from build123d import *

# Parameters (mm, degrees)
F1_DEPTH = 25.4
F3_DEPTH = 12.7
F4_W     = 5.8812871575
F4_H     = 48.275558278
F4_W_2   = 5.8812852949
F5_DEPTH = 1.27
F7_DEPTH = 1.27


with BuildPart() as f1:
    # F0 (on Front) → F1 (new body)
    with BuildSketch(Plane.XZ):
        with BuildLine():
            Line((-42.643032968, 37.9803813994), (-42.643032968, 0))
            Line((-42.643032968, 0), (0, 0))
            Line((0, 0), (42.642146349, 0))
            Line((42.642146349, 0), (42.642146349, 37.9803813994))
            ThreePointArc((42.642146349, 37.9803813994), (-0.0004433095, 75.7243208105), (-42.643032968, 37.9803813994))
        make_face()
        Polygon((0, 0), (-42.643032968, 0), (-42.643032968, -75.733192265), (42.642146349, -75.733192265), (42.642146349, 0), align=None)
    extrude(amount=F1_DEPTH)

    # F2 (on face) → F3 (join)
    with BuildSketch(Plane(origin=(0, 0, 0), x_dir=(-1, 0, 0), z_dir=(0, 1, 0))):
        with BuildLine():
            ThreePointArc((42.643032968, 37.9803813994), (0.0004433095, 75.4104343916), (-42.642146349, 37.9803813994))
            Line((-42.642146349, 37.9803813994), (-42.642146349, -75.733192265))
            Line((-42.642146349, -75.733192265), (42.643032968, -75.733192265))
            Line((42.643032968, -75.733192265), (42.643032968, 37.9803813994))
        make_face()
    extrude(amount=F3_DEPTH)

    # F4 (on face) → F5 (join)
    with BuildSketch(Plane.XZ.offset(25.4)):
        with Locations((-30.264120549, -9.6796164289)):
            Rectangle(F4_W, F4_H)
        with Locations((30.0190644339, -9.6796164289)):
            Rectangle(F4_W_2, F4_H)
    extrude(amount=F5_DEPTH)

    # F6 (on face) → F7 (join)
    with BuildSketch(Plane.XZ.offset(25.4)):
        with BuildLine():
            ThreePointArc((27.0784217864, 37.9803813994), (-0.1225275919, 61.2469587983), (-27.3234769702, 37.9803813994))
            Line((-27.3234769702, 37.9803813994), (27.0784217864, 37.9803813994))
        make_face()
    extrude(amount=F7_DEPTH)


solid = f1.part
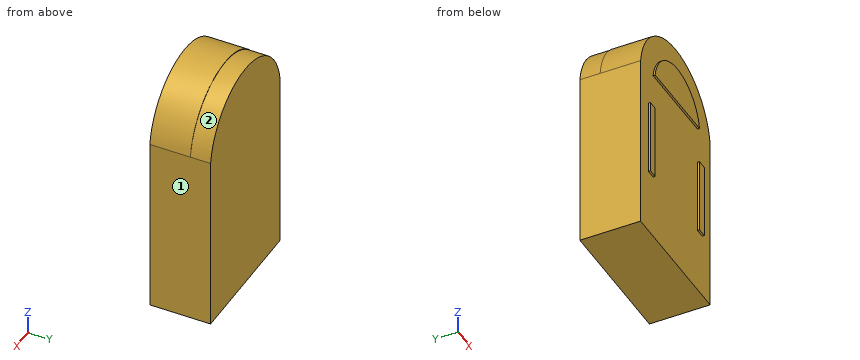
Source: CAD feature listing. Evaluate the final solid. Frame: model axes, mm. Face numbers are marked on the shaded views. A direction names the side the tool comes from. Round coordinates to 2 decimals unless told otherwise and drop trailing zeros. Loops run counter-clockwise (first coordinate to the right, second up) from the corner with the lowest first, then second, coordinate; pieces in that order, holes last. Notation, with made-up numbers: (15, 77) - (57, 77) arc R21 ccw to (57, 114) - close; hole circle Ø5 at (83, 28). An arc over 180 degrees is marked (long way). Write item = value, one per line. Start each with the question number.
(1) Section query D-D, the plane z = 55. Output: boundary loops of the cut face in (x, y).
(2) Ray query, line 1 along Y through (x, z) = (-6.5, 27); line 2 along Z through (x, y) = (-34, -20.5); line 3 along Z through (x, y) = (-26.5, -21). Return the intervals inside material, ascending. Write a range as from..to.
(3) Set-up query: the marked faces 1 and 2. Return all of +Z, -Z, +X, -X, +Y, -Y with unobstructed straight access to the full face (end or side cutting, diameter ignored); none if empty.
(4) Section query B-B, the plane x = -23.5. Output: boundary loops of the cut face in (y, z).
(5) Section query C-C, the plane y = -16.5. Output: boundary loops of the cut face in (x, z), plus the area to 3 significant figures.
(6) Pin query (flat end, axial travel): pin 1 (1 mm diameter, centred on x = 31, y = -26, fed in from -Z); pin 2 (0.6 mm diameter, centred on y = -26, z = -17, fed in from +X); pin 3 (2 mm diameter, centred on x = 20.5, z = -21, fed in from -Y). Return the tip coordinate at first contact, or that it passes through.
(7) Section query A-A, the plane z = 0.5. Output: boundary loops of the cut face in (x, y).
Conclusion:
q1.outline = (-36.76, -25.4) - (-17.59, -25.4) - (-17.59, -26.67) - (17.34, -26.67) - (17.34, -25.4) - (36.76, -25.4) - (36.76, 0) - (36.59, 0) - (36.59, 12.7) - (-36.59, 12.7) - (-36.59, 0) - (-36.76, 0) - close
q2.line_1 = -25.4..12.7
q2.line_2 = -75.73..59.02
q2.line_3 = -75.73..66.58
q3.face_1 = +Z, -Z, +X, +Y, -Y
q3.face_2 = +Z, +Y
q4.outline = (-26.67, 37.98) - (-25.4, 37.98) - (-25.4, -75.73) - (12.7, -75.73) - (12.7, 68.42) - (0, 68.42) - (0, 68.73) - (-25.4, 68.73) - (-25.4, 48.26) - (-26.67, 48.26) - close
q5.outline = (-42.64, -75.73) - (42.64, -75.73) - (42.64, 37.98) arc R42.96 ccw to (-42.64, 37.98) - close
q5.area = 12,200 mm2
q6.pin_1 = -33.82
q6.pin_2 = 32.96
q6.pin_3 = -25.4
q7.outline = (-42.64, -25.4) - (-33.2, -25.4) - (-33.2, -26.67) - (-27.32, -26.67) - (-27.32, -25.4) - (27.08, -25.4) - (27.08, -26.67) - (32.96, -26.67) - (32.96, -25.4) - (42.64, -25.4) - (42.64, 12.7) - (-42.64, 12.7) - close
